Verification items for the finished model (mm, model axes). A direction names the side the tool comes from. Give positions to 0.01 mm unless a question says otherwise; leave off trailing zeros. Loops run counter-clockwise (first coordinate to the right, second up) from the corner with the lowest first, then second, coordinate; pieces in that order, holes last. Notation, with made-up numbers: (20.25, 69) - (46.25, 69) arc R19 cw to (46.25, 90) - close; hole circle Ø9 at (-9.75, 30). An arc over 180 degrees is marked (long way). One line per question, with ' | ' between items. Start each with the question number.
1. Mould release check, pull along Y, two halves, no side actions. Record for faces 1 (the face through (-16.637, 0, 225)), 2 (the face through (0, 19.05, 225)), 3 (the face through (19.05, 0, 225)), 4 (the face through (0, -19.05, 225)): +Y half, -Y half, draft (parallel to the pull), parting line (faces both ways), or undercut.
2. Section check B-B, the plane z = 19.05. Enter the section's corners in (x, y).
3. Tool access check on faces 5 (the face through (0, 16.637, 225)), 6 (the face through (-2.93, -17.83, 32.22)). Record the directions out of +Z, -Z, +X, -X, +Y, -Y that give a thin tool (end or side, any length) a straight path to the whole face; none if there is none.
4. Thickness scan on line 1 along Y through (x, z) = (13.5, 20.5); line 2 along Z through (x, y) = (0, -17.85). Record the ranges inside material, lowest first. Write a range as from..to.
5. Section check D-D, the plane z = 317.5. Enter the section's corners in (x, y), then the cut area to 3 significant figures.
6. Section check C-C, the plane y = 0.5. Enter the section's corners in (x, z).
7. Section check A-A, the plane x = 0. Enter the section's corners in (y, z).
from build123d import *

# Parameters (mm, degrees)
BOSS_EXTRUDE1_DEPTH = 457.2
SKETCH2_R           = 13.49375
CUT_EXTRUDE1_DEPTH  = 228.6


with BuildPart() as part:
    # Sketch1 → Boss-Extrude1 (new body)
    with BuildSketch(Plane.XY):
        with BuildLine():
            Line((-16.637, -19.05), (16.637, -19.05))
            ThreePointArc((16.637, -19.05), (18.343248663, -18.343248663), (19.05, -16.637))
            Line((19.05, -16.637), (19.05, 16.637))
            ThreePointArc((19.05, 16.637), (18.343248663, 18.343248663), (16.637, 19.05))
            Line((16.637, 19.05), (-16.637, 19.05))
            ThreePointArc((-16.637, 19.05), (-18.343248663, 18.343248663), (-19.05, 16.637))
            Line((-19.05, 16.637), (-19.05, -16.637))
            ThreePointArc((-19.05, -16.637), (-18.343248663, -18.343248663), (-16.637, -19.05))
        make_face()
        with BuildLine():
            Line((-14.224, -16.637), (14.224, -16.637))
            ThreePointArc((14.224, -16.637), (15.930248663, -15.930248663), (16.637, -14.224))
            Line((16.637, -14.224), (16.637, 14.224))
            ThreePointArc((16.637, 14.224), (15.930248663, 15.930248663), (14.224, 16.637))
            Line((14.224, 16.637), (-14.224, 16.637))
            ThreePointArc((-14.224, 16.637), (-15.930248663, 15.930248663), (-16.637, 14.224))
            Line((-16.637, 14.224), (-16.637, -14.224))
            ThreePointArc((-16.637, -14.224), (-15.930248663, -15.930248663), (-14.224, -16.637))
        make_face(mode=Mode.SUBTRACT)
    extrude(amount=BOSS_EXTRUDE1_DEPTH)

    # Sketch2 → Cut-Extrude1 (cut, symmetric)
    with BuildSketch(Plane(origin=(0, 0, 0), x_dir=(1, 0, 0), z_dir=(0, 1, 0))):
        with Locations((0, -19.05)):
            Circle(SKETCH2_R)
    extrude(amount=CUT_EXTRUDE1_DEPTH, both=True, mode=Mode.SUBTRACT)


solid = part.part
Results list:
1) face 1: undercut | face 2: +Y half | face 3: draft | face 4: -Y half
2) outline: (-19.05, -16.64) arc R2.41 ccw to (-16.64, -19.05) - (-13.49, -19.05) - (-13.49, -16.64) - (-14.22, -16.64) arc R2.41 cw to (-16.64, -14.22) - (-16.64, 14.22) arc R2.41 cw to (-14.22, 16.64) - (-13.49, 16.64) - (-13.49, 19.05) - (-16.64, 19.05) arc R2.41 ccw to (-19.05, 16.64) - close; (13.49, -19.05) - (16.64, -19.05) arc R2.41 ccw to (19.05, -16.64) - (19.05, 16.64) arc R2.41 ccw to (16.64, 19.05) - (13.49, 19.05) - (13.49, 16.64) - (14.22, 16.64) arc R2.41 cw to (16.64, 14.22) - (16.64, -14.22) arc R2.41 cw to (14.22, -16.64) - (13.49, -16.64) - close
3) face 5: +Z, -Z | face 6: +Y, -Y
4) line 1: -19.05..-16.64, 16.64..19.05 | line 2: 0..5.56, 32.54..457.2
5) outline: (-19.05, -16.64) arc R2.41 ccw to (-16.64, -19.05) - (16.64, -19.05) arc R2.41 ccw to (19.05, -16.64) - (19.05, 16.64) arc R2.41 ccw to (16.64, 19.05) - (-16.64, 19.05) arc R2.41 ccw to (-19.05, 16.64) - close; hole (-16.64, -14.22) arc R2.41 ccw to (-14.22, -16.64) - (14.22, -16.64) arc R2.41 ccw to (16.64, -14.22) - (16.64, 14.22) arc R2.41 ccw to (14.22, 16.64) - (-14.22, 16.64) arc R2.41 ccw to (-16.64, 14.22) - close | area: 344 mm²
6) outline: (-19.05, 0) - (-16.64, 0) - (-16.64, 457.2) - (-19.05, 457.2) - close; (16.64, 0) - (19.05, 0) - (19.05, 457.2) - (16.64, 457.2) - close
7) outline: (-19.05, 0) - (-16.64, 0) - (-16.64, 5.56) - (-19.05, 5.56) - close; (-19.05, 32.54) - (-16.64, 32.54) - (-16.64, 457.2) - (-19.05, 457.2) - close; (16.64, 0) - (19.05, 0) - (19.05, 5.56) - (16.64, 5.56) - close; (16.64, 32.54) - (19.05, 32.54) - (19.05, 457.2) - (16.64, 457.2) - close
